Design review of the part shown in the three views and the two pictorial views. Dimensions are in mm from the part's minimum x, y and z. Coordinates: 2 decimals unless noted, no trailing zeros. Loops run counter-clockwise (first coordinate to the right, second up) from the corner with the lowest first, then second, coordinate; pieces in that order, holes last. Notation, with made-up numbers: M 28,48 L 84,48 A19 ccw 84,64 Z; hole C 28,-34.5 d5. An arc over 180 degrees is marked long. Answer as a JSON object with one key per item and string values. Group by question number.
Item 1: Add section D-D (z = 49). State the section outline as (x, y) points (1 decimal).
Item 2: Mouldability with a two-part tool opening along Y and no side actions: class the marked faces 1, 2 and 3 as +Y half, -Y half, draft (parallel to the pull), parting line (faces both ways), or undercut.
Item 3: Add section C-C (y = 6). State the section outline as (x, z) points.
Item 4: Add section A-A (x = 30). State the section outline as (y, z) points, then the cut area to 3 significant figures.
Item 5: Insertion check: pin 1 (1.5 mm diameter, centred on x = 19, y = 4.5, fed in from -Z) (1 decimal); pin 2 (5 mm diameter, centred on y = 2, z = 25, fed in from -X); pin 3 (2 mm diameter, centred on y = 2.5, z = 21.5, fed in from +X). Each pin has a flat end and moves straight along its axis. Give the tip position at first contact, or say it passes through.
Item 6: Add section B-B (z = 30). State the section outline as (x, y) points (1 decimal), then the cut area to 3 significant figures.
Item 7: Wall thickness on L1, parallel to Y at x = 20.25, z = 30; L2, parallel to Z at x = 48.5, y = 8.75; L3, parallel to Z at x = 50, y = 1.5 (1 decimal): over which ranges is each line inside the solid? List them lowest first. Write a range as from..to.
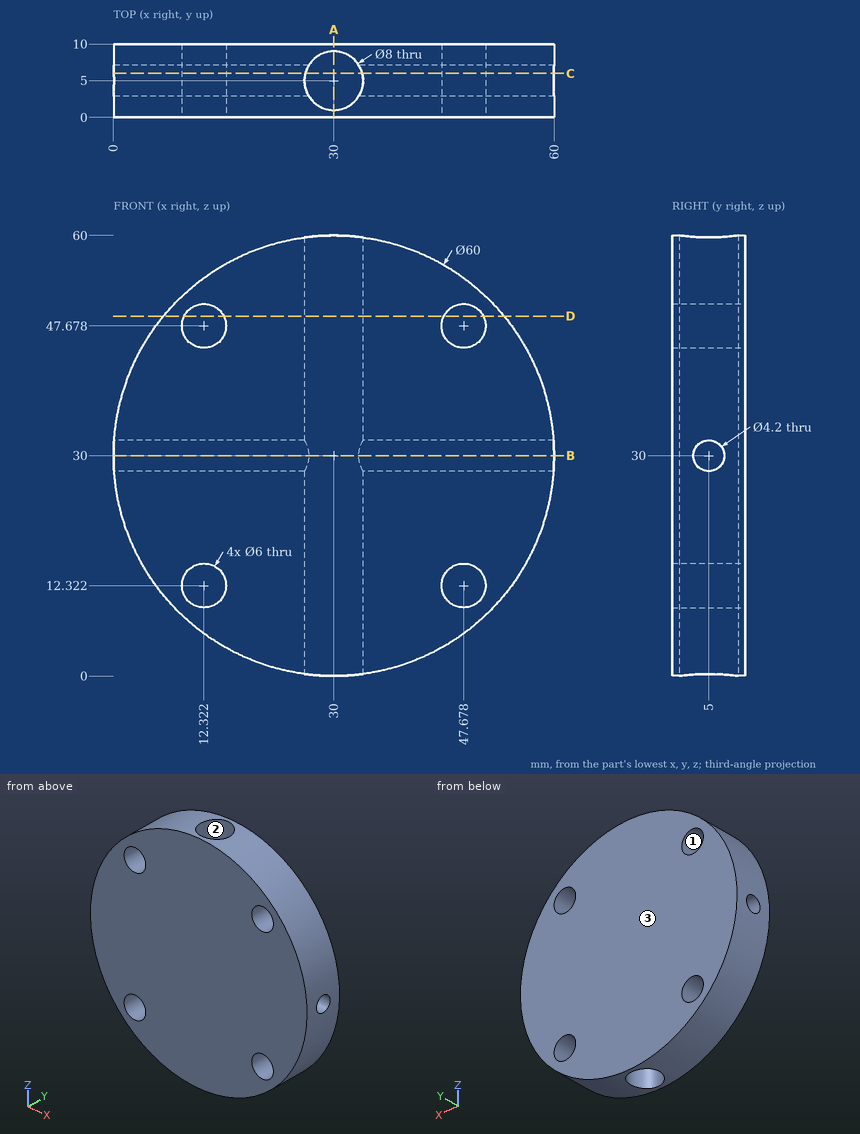
From the geometry:
{
 "1": {"outline": "M 6.8,0 L 9.6,0 L 9.6,10 L 6.8,10 Z; M 15,0 L 45,0 L 45,10 L 15,10 Z; M 50.4,0 L 53.2,0 L 53.2,10 L 50.4,10 Z; hole C 30,5 d8"},
 "2": {"face 1": "draft", "face 2": "undercut", "face 3": "+Y half"},
 "3": {"outline": "M 0.06,28.15 A30 ccw 26.13,0.25 L 26.13,28.15 Z; M 0.06,31.85 L 26.13,31.85 L 26.13,59.75 A30 ccw Z; M 33.87,0.25 A30 ccw 59.94,28.15 L 33.87,28.15 Z; M 33.87,31.85 L 59.94,31.85 A30 ccw 33.87,59.75 Z; hole C 12.32,12.32 d6; hole C 12.32,47.68 d6; hole C 47.68,12.32 d6; hole C 47.68,47.68 d6"},
 "4": {"outline": "M 0,0 L 1,0 L 1,60 L 0,60 Z; M 9,0 L 10,0 L 10,60 L 9,60 Z", "area": "120 mm²"},
 "5": {"pin 1": "stops at z = 1.8", "pin 2": "stops at x = 0.1", "pin 3": "stops at x = 59.05"},
 "6": {"outline": "M 0,0 L 60,0 L 60,2.9 L 33.4,2.9 A4 cw 26.6,2.9 L 0,2.9 Z; M 0,7.1 L 26.6,7.1 A4 cw 33.4,7.1 L 60,7.1 L 60,10 L 0,10 Z", "area": "330 mm²"},
 "7": {"L1": "y = 0..2.9, 7.1..10", "L2": "z = 6.38..9.44, 15.21..44.79, 50.56..53.62", "L3": "z = 7.6..10.4, 14.2..45.8, 49.6..52.4"}
}
